Verification items for this drawing (mm, ordinates from the low corner). Coordinates: 2 decimals unless noted, no trailing zeros. Order: outer loops, then holes, each group sorted by start corner. A loop starts at its lowest first (then second) coordinate and runs counter-clockwise, first axis right, second up. Notation, with made-up numbers: M -12,65 L 14,65 A17 cw 14,81 Z; hole C 77,-12.5 d11. An arc over 180 degrees is marked long. One line per item, written item: value. Start each with the question number.
1) Go/stop test with a flat-tipped pin: P1, Ø3, axis at x = 7, y = 2, coming from the -Z side. Record where the tip stops, or that it passes through.
2) Sectioned sample at D-D, the plane z = 7. Enter the section's corners in (x, y).
3) Sectioned sample at C-C, the plane y = 1.5. Enter the section's corners in (x, z).
4) Sectioned sample at A-A, the plane z = 67.5. Enter the section's corners in (x, y).
5) Thickness scan on L1, parallel to Z at x = 4.5, y = 1.65; L2, parallel to X at y = 1.8, z = 67.5; L3, parallel to Z at x = 3.75, y = 0.3. Record the ranges inside material, lowest first. Write a range as from..to.
6) Sectioned sample at B-B, the plane x = 4.5. Enter the section's corners in (y, z).
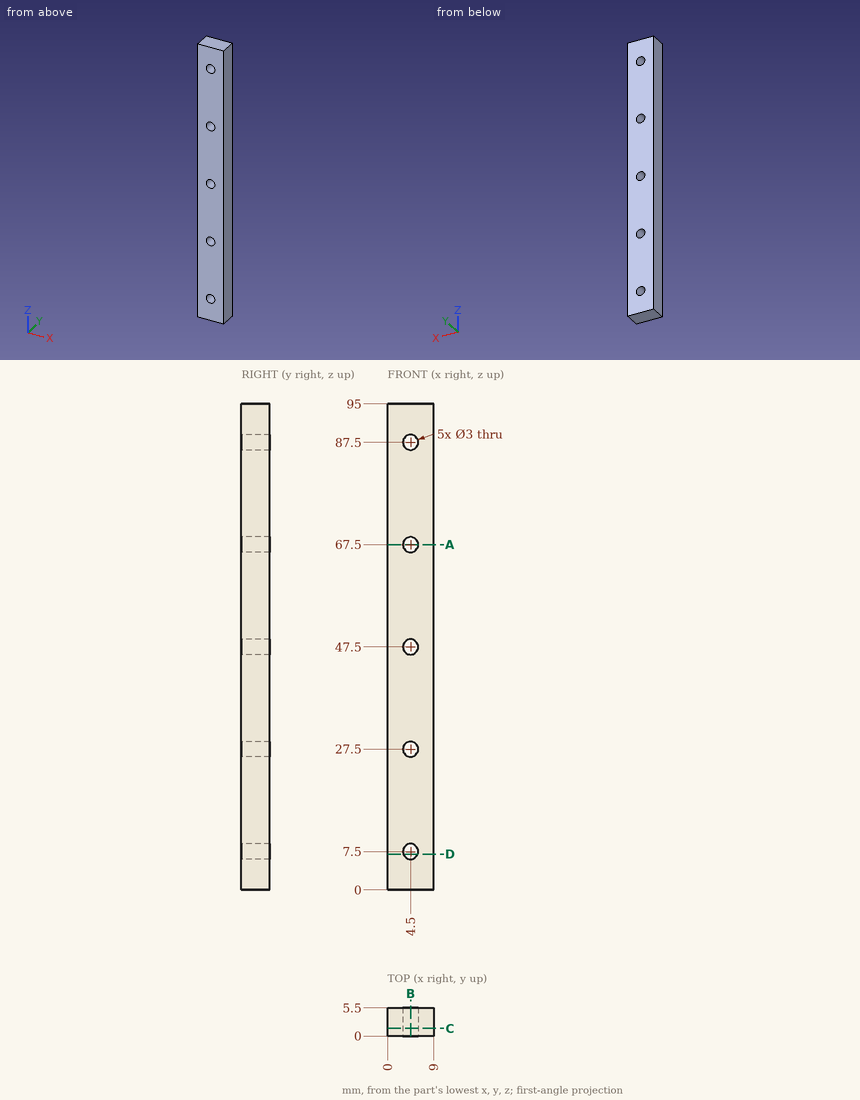
Final values:
1. P1: stops at z = 0
2. outline: M 0,0 L 3.09,0 L 3.09,5.5 L 0,5.5 Z; M 5.91,0 L 9,0 L 9,5.5 L 5.91,5.5 Z
3. outline: M 0,0 L 9,0 L 9,95 L 0,95 Z; hole C 4.5,7.5 d3; hole C 4.5,27.5 d3; hole C 4.5,47.5 d3; hole C 4.5,67.5 d3; hole C 4.5,87.5 d3
4. outline: M 0,0 L 3,0 L 3,5.5 L 0,5.5 Z; M 6,0 L 9,0 L 9,5.5 L 6,5.5 Z
5. L1: z = 0..6, 9..26, 29..46, 49..66, 69..86, 89..95
5. L2: x = 0..3, 6..9
5. L3: z = 0..6.2, 8.8..26.2, 28.8..46.2, 48.8..66.2, 68.8..86.2, 88.8..95
6. outline: M 0,0 L 5.5,0 L 5.5,6 L 0,6 Z; M 0,9 L 5.5,9 L 5.5,26 L 0,26 Z; M 0,29 L 5.5,29 L 5.5,46 L 0,46 Z; M 0,49 L 5.5,49 L 5.5,66 L 0,66 Z; M 0,69 L 5.5,69 L 5.5,86 L 0,86 Z; M 0,89 L 5.5,89 L 5.5,95 L 0,95 Z
